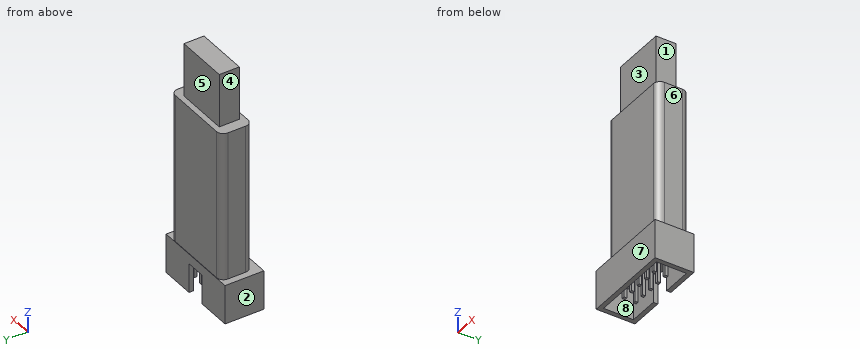
from build123d import *

# Parameters (mm, degrees)
SKETCH1_W           = 12
SKETCH1_H           = 4.5
BOSS_EXTRUDE1_DEPTH = 12
SKETCH2_W           = 17
SKETCH2_H           = 7
BOSS_EXTRUDE2_DEPTH = 33.5
SKETCH3_W           = 20
SKETCH3_H           = 8.7
BOSS_EXTRUDE3_DEPTH = 8.8
SKETCH4_W           = 18
SKETCH4_H           = 6.7
SKETCH4_W_2         = 4.5
SKETCH4_H_2         = 1
CUT_EXTRUDE2_DEPTH  = 6.6
SKETCH5_W           = 0.65
SKETCH5_H           = 0.65
BOSS_EXTRUDE4_DEPTH = 5.8
LPATTERN1_COUNT     = 3
LPATTERN1_PITCH     = 2.54
LPATTERN1_COL_COUNT = 3
LPATTERN1_COL_PITCH = 2.54
FILLET1_R           = 1.5


with BuildPart() as part:
    # Sketch1 → Boss-Extrude1 (new body)
    with BuildSketch(Plane.XY):
        Rectangle(SKETCH1_W, SKETCH1_H)
    extrude(amount=-BOSS_EXTRUDE1_DEPTH)

    # Sketch2 → Boss-Extrude2 (add)
    with BuildSketch(Plane(origin=(0, 0, -12), x_dir=(-1, 0, 0), z_dir=(0, 0, -1))):
        Rectangle(SKETCH2_W, SKETCH2_H)
    extrude(amount=BOSS_EXTRUDE2_DEPTH)

    # Sketch3 → Boss-Extrude3 (add)
    with BuildSketch(Plane(origin=(0, 0, -45.5), x_dir=(-1, 0, 0), z_dir=(0, 0, -1))):
        with Locations((0, -0.75)):
            Rectangle(SKETCH3_W, SKETCH3_H)
    extrude(amount=BOSS_EXTRUDE3_DEPTH)

    # Sketch4 → Cut-Extrude2 (cut)
    with BuildSketch(Plane(origin=(0, 0, -54.3), x_dir=(-1, 0, 0), z_dir=(0, 0, -1))):
        with Locations((0, -0.75)):
            Rectangle(SKETCH4_W, SKETCH4_H)
        with Locations((0, 3.1)):
            Rectangle(SKETCH4_W_2, SKETCH4_H_2)
    extrude(amount=-CUT_EXTRUDE2_DEPTH, mode=Mode.SUBTRACT)

    # Sketch5 → Boss-Extrude4 (add)
    with BuildSketch(Plane(origin=(0, 0, -47.7), x_dir=(-1, 0, 0), z_dir=(0, 0, -1))):
        with Locations((0, 0.52)):
            Rectangle(SKETCH5_W, SKETCH5_H)
        with Locations((0, -2.02)):
            Rectangle(SKETCH5_W, SKETCH5_H)
    boss_extrude4 = extrude(amount=BOSS_EXTRUDE4_DEPTH)

    # LPattern1: Boss-Extrude4 ×3
    with Locations(*[(i * LPATTERN1_PITCH, 0, 0) for i in range(1, LPATTERN1_COUNT)]):
        add(boss_extrude4)

    # LPattern1 col: Boss-Extrude4 ×3
    with Locations(*[(-i * LPATTERN1_COL_PITCH, 0, 0) for i in range(1, LPATTERN1_COL_COUNT)]):
        add(boss_extrude4)

    # Fillet1
    fillet1_edges = [part.edges().sort_by_distance(p)[0] for p in [
        (8.5, 3.5, -28.75),
        (8.5, -3.5, -28.75),
        (-8.5, -3.5, -28.75),
        (-8.5, 3.5, -28.75),
    ]]
    fillet(fillet1_edges, radius=FILLET1_R)


solid = part.part
Geometry: final body of the model. Coordinates: model frame, mm. Face numbers are marked on the shaded views. A direction names the side the tool comes from. Give positions to 0.01 mm unless a question says otherwise; leave off trailing zeros. Write each loop counter-clockwise with the first axis right and the second up, starting at its lowest first coordinate (ties: lowest second). Pieces come first, ordered by that corner, then holes.
(1) First-contact query: P1, Ø6, axis at x = 0.5, z = -14, coming from the -Y side; P2, Ø2, axis at y = -4, z = -19.5, coming from the +X side; P3, Ø12, axis at x = -7, z = -32.5, coming from the +Y side. Flat tips, straight axial feed; report the tip coordinate or a pass-through.
(2) Cut plane B-B, the plane x = -1.5. Return loops of the section in (y, z), then the cut area to 3 significant figures.
(3) Mould query, pull axis Y, two halves, no side actions, for the marked faces 6, 7 and 8. Classes: released by +Y, released by -Y, zero draft, split by the parting line, or undercut.
(4) Ray query, line 1 (Y direction, x = 8.75, z = -49.5); line 2 (Y direction, x = 2.75, z = -48) (3 decimals); line 3 (X direction, y = -0.75, z = -50). Return the intervals inside material, ascending.
(5) Cut plane C-C, the plane z = -40.5. Return loops of the section in (x, y).
(6) Access query for the marked faces 1, 2, 3, 4 and 5. Directions: +Z, -Z, +X, -X, +Y, -Y. A direction counts if a zero-diameter tool reaches every point of the face in a straight line with its end or side. Return the directions, or none.
(7) Cut plane A-A, the plane y = -1. Return loops of the section in (x, z).
(8) Cut plane D-D, the plane x = -8. Return loops of the section in (y, z).
Values follow:
1. P1: stops at y = -3.5
1. P2: stops at x = 8.12
1. P3: stops at y = 3.5
2. outline: (-5.1, -54.3) - (-4.1, -54.3) - (-4.1, -47.7) - (3.6, -47.7) - (3.6, -45.5) - (3.5, -45.5) - (3.5, -12) - (2.25, -12) - (2.25, 0) - (-2.25, 0) - (-2.25, -12) - (-3.5, -12) - (-3.5, -45.5) - (-5.1, -45.5) - close
2. area: 314 mm2
3. face 6: zero draft
3. face 7: released by -Y
3. face 8: undercut
4. line 1: y = -5.1 to -4.1, 2.6 to 3.6
4. line 2: y = -5.1 to -4.1, -2.345 to -1.695, 0.195 to 0.845, 2.6 to 3.6
4. line 3: x = -10 to -9, 9 to 10
5. outline: (-8.5, -2) arc R1.5 ccw to (-7, -3.5) - (7, -3.5) arc R1.5 ccw to (8.5, -2) - (8.5, 2) arc R1.5 ccw to (7, 3.5) - (-7, 3.5) arc R1.5 ccw to (-8.5, 2) - close
6. face 1: +Z, +X, +Y, -Y
6. face 2: +Z, -Z, -X, +Y, -Y
6. face 3: +Z, +X, -X, -Y
6. face 4: +Z, -X, +Y, -Y
6. face 5: +Z, +X, -X, +Y
7. outline: (-10, -54.3) - (-9, -54.3) - (-9, -47.7) - (9, -47.7) - (9, -54.3) - (10, -54.3) - (10, -45.5) - (8.5, -45.5) - (8.5, -12) - (6, -12) - (6, 0) - (-6, 0) - (-6, -12) - (-8.5, -12) - (-8.5, -45.5) - (-10, -45.5) - close
8. outline: (-5.1, -54.3) - (-4.1, -54.3) - (-4.1, -47.7) - (2.6, -47.7) - (2.6, -54.3) - (3.6, -54.3) - (3.6, -45.5) - (3.12, -45.5) - (3.12, -12) - (-3.12, -12) - (-3.12, -45.5) - (-5.1, -45.5) - close
